from build123d import *

# Parameters (mm, degrees)
CROQUIS1_R              = 1.5
CROQUIS1_R_2            = 2.5
SALIENTE_EXTRUIR1_DEPTH = 3
CROQUIS2_R              = 1.5
CORTAR_EXTRUIR1_DEPTH   = 10
CROQUIS4_R              = 1.5
CORTAR_EXTRUIR2_DEPTH   = 10
CROQUIS6_R              = 1.75
CORTAR_EXTRUIR4_DEPTH   = 181.797465623
CROQUIS7_R              = 1.5
CORTAR_EXTRUIR5_DEPTH   = 10


with BuildPart() as part:
    # Croquis1 → Saliente-Extruir1 (new body)
    with BuildSketch(Plane(origin=(0, 0, 0), x_dir=(1, 0, 0), z_dir=(0, 1, 0))):
        with BuildLine():
            Line((-50, -50), (29, -50))
            ThreePointArc((29, -50), (45.026638216, -44.431709815), (56.55148357, -31.980327255))
            ThreePointArc((56.55148357, -31.980327255), (65.032402177, -23.219540774), (76.793010893, -20))
            ThreePointArc((76.793010893, -20), (87.064733458, -28.647586327), (90, -41.75))
            ThreePointArc((90, -41.75), (100, -51.75), (110, -41.75))
            ThreePointArc((110, -41.75), (112.935266542, -28.647586327), (123.206989107, -20))
            Line((123.206989107, -20), (170.206989107, -20))
            ThreePointArc((170.206989107, -20), (172.328309451, -19.121320344), (173.206989107, -17))
            Line((173.206989107, -17), (173.206989107, 17))
            ThreePointArc((173.206989107, 17), (172.328309451, 19.121320344), (170.206989107, 20))
            Line((170.206989107, 20), (123.206989107, 20))
            ThreePointArc((123.206989107, 20), (112.935266542, 28.647586327), (110, 41.75))
            ThreePointArc((110, 41.75), (100, 51.75), (90, 41.75))
            ThreePointArc((90, 41.75), (87.064733458, 28.647586327), (76.793010893, 20))
            ThreePointArc((76.793010893, 20), (65.032402177, 23.219540774), (56.55148357, 31.980327255))
            ThreePointArc((56.55148357, 31.980327255), (45.026638216, 44.431709815), (29, 50))
            Line((29, 50), (-50, 50))
            Line((-50, 50), (-50, 15))
            Line((-50, 15), (-75, 15))
            Line((-75, 15), (-75, -15))
            Line((-75, -15), (-50, -15))
            Line((-50, -15), (-50, -50))
        make_face()
        with Locations(Location((-29, -24.5, 0), (0, 0, 270))):
            Circle(CROQUIS1_R, mode=Mode.SUBTRACT)
        with Locations(Location((29, -24.5, 0), (0, 0, 270))):
            Circle(CROQUIS1_R, mode=Mode.SUBTRACT)
        with Locations(Location((100, -41.75, 0), (0, 0, 270))):
            Circle(CROQUIS1_R_2, mode=Mode.SUBTRACT)
        with Locations(Location((-29, 24.5, 0), (0, 0, 270))):
            Circle(CROQUIS1_R, mode=Mode.SUBTRACT)
        with Locations(Location((29, 24.5, 0), (0, 0, 270))):
            Circle(CROQUIS1_R, mode=Mode.SUBTRACT)
        with Locations(Location((100, 41.75, 0), (0, 0, 270))):
            Circle(CROQUIS1_R_2, mode=Mode.SUBTRACT)
    extrude(amount=SALIENTE_EXTRUIR1_DEPTH)

    # Croquis2 → Cortar-Extruir1 (cut)
    with BuildSketch(Plane.XZ):
        with Locations(Location((-72, 9.943892899, 0), (0, 0, 270))):
            Circle(CROQUIS2_R)
        with Locations(Location((-48, 9.943892899, 0), (0, 0, 270))):
            Circle(CROQUIS2_R)
        with Locations(Location((-72, -10.056107101, 0), (0, 0, 270))):
            Circle(CROQUIS2_R)
        with Locations(Location((-48, -10.056107101, 0), (0, 0, 270))):
            Circle(CROQUIS2_R)
    extrude(amount=-CORTAR_EXTRUIR1_DEPTH, mode=Mode.SUBTRACT)

    # Croquis4 → Cortar-Extruir2 (cut)
    with BuildSketch(Plane.XZ):
        with Locations(Location((-25, 46, 0), (0, 0, 270))):
            Circle(CROQUIS4_R)
        with Locations(Location((25, 46, 0), (0, 0, 270))):
            Circle(CROQUIS4_R)
        with Locations(Location((119.206989107, 16, 0), (0, 0, 270))):
            Circle(CROQUIS4_R)
        with Locations(Location((169.206989107, 16, 0), (0, 0, 270))):
            Circle(CROQUIS4_R)
        with Locations(Location((169.206989107, -16, 0), (0, 0, 90))):
            Circle(CROQUIS4_R)
        with Locations(Location((119.206989107, -16, 0), (0, 0, 90))):
            Circle(CROQUIS4_R)
        with Locations(Location((25, -46, 0), (0, 0, 90))):
            Circle(CROQUIS4_R)
        with Locations(Location((-25, -46, 0), (0, 0, 90))):
            Circle(CROQUIS4_R)
    extrude(amount=-CORTAR_EXTRUIR2_DEPTH, mode=Mode.SUBTRACT)

    # Croquis6 → Cortar-Extruir4 (cut, through all)
    with BuildSketch(Plane(origin=(0, 3, 0), x_dir=(1, 0, 0), z_dir=(0, 1, 0))):
        with Locations(Location((101.826339239, -24.115973685, 0), (0, 0, 270))):
            Circle(CROQUIS6_R)
        with Locations(Location((101.373426984, 14.680198998, 0), (0, 0, 270))):
            Circle(CROQUIS6_R)
    extrude(amount=-CORTAR_EXTRUIR4_DEPTH, mode=Mode.SUBTRACT)

    # Croquis7 → Cortar-Extruir5 (cut)
    with BuildSketch(Plane.XZ):
        with Locations(Location((93.500729234, -41.847362769, 0), (0, 0, 270))):
            Circle(CROQUIS7_R)
        with Locations(Location((106.499270766, -41.652637231, 0), (0, 0, 270))):
            Circle(CROQUIS7_R)
        with Locations(Location((93.500127651, 41.709263638, 0), (0, 0, 270))):
            Circle(CROQUIS7_R)
        with Locations(Location((106.499872349, 41.790736362, 0), (0, 0, 270))):
            Circle(CROQUIS7_R)
    extrude(amount=-CORTAR_EXTRUIR5_DEPTH, mode=Mode.SUBTRACT)


solid = part.part
Build history of the part. All positions in model axes, mm. A direction names the side the tool comes from. Give positions to 0.01 mm unless a question says otherwise; leave off trailing zeros. Use one line per item in the form item = value.
1) Drop flat-ended pins along their axis: pin 1 (4 mm diameter, centred on x = -48, z = -10.06, fed in from +Y); pin 2 (0.9 mm diameter, centred on x = -21.5, y = 1, fed in from -Z); pin 3 (1.5 mm diameter, centred on y = 2, z = 19, fed in from -X); pin 4 (12 mm diameter, centred on x = 119, z = 39, fed in from -Y). Give the stop position or say it passes through.
Calculated:
pin_1 = 3
pin_2 = -50
pin_3 = -50
pin_4 = through
2) Probe probe 1 along Z at (x, y) = (145, 2.6); probe 2 along Z at (x, y) = (-21, 1.25); probe 3 along X at (y, z) = (0.5, 35.5). List the from-to ranges inside material, lowest first.
Calculated:
probe_1 = -20 to 20
probe_2 = -50 to 50
probe_3 = -50 to 54.34, 89.72 to 110.28
3) Tool access for faces 5 (the face through (45.23, 1.48, -44.3)), 6 (the face through (44.83, 1.48, 44.56)), 7 (the face through (47, 0, -1)): list every direction of +Z, -Z, +X, -X, +Y, -Y with a clear straight run to the whole face (end or side of a thin tool).
Calculated:
face_5 = -Z, +Y, -Y
face_6 = +Z, +Y, -Y
face_7 = +Z, -Z, +X, -X, -Y
4) Saw through at A-A (y = 1.75). State how many separate pieces and enclosed holes the cut face has, plus the area to 3 significant figures.
Calculated:
separate_pieces = 1
enclosed_holes = 24
area = 17,200 mm2
5) Two-plate mould, pull along Z, no slides. Class faces 1 (the face through (99.78, 1.479, 51.748)), 2 (the face through (102.11, 1.48, -40.41)), 3 (the face through (47, 3, -1)), 4 (the face through (102.48, 1.48, 41.42)): released by +Z, released by -Z, zero draft, split by the parting line, or undercut.
Calculated:
face_1 = released by +Z
face_2 = undercut
face_3 = zero draft
face_4 = undercut
